Input: part model. Units: mm. Frame: model coordinates. Round coordinates to 2 decimals unless told otherwise and drop trailing zeros. Order: outer loops, then holes, each group sorted by start corner. A loop starts at its lowest first (then second) coordinate and runs counter-clockwise, first axis right, second up. Notation, with made-up numbers: (-9, -4.5) -> (13, -4.5) arc R35 ccw to (13, 32.5) -> close; hole circle Ø5 at (-17, -9.5). An arc over 180 degrees is marked (long way). Answer as CSV lines item,"result". Start each with the question number.
1) Section query C-C, the plane x = 17.5. Output: boundary loops of the cut face in (y, z), and give its area (3 significant figures).
2) Section query B-B, the plane z = 3.2. Output: boundary loops of the cut face in (x, y) (3 decimals).
3) Section query A-A, the plane y = -8.3. Output: boundary loops of the cut face in (x, z), and give its area (3 significant figures).
4) Line query: L1, parallel to Y at x = -12, z = 2.5; L2, parallel to Y at x = 15, z = 3.2; L3, parallel to X at y = 14.5, z = 1.3. Output: solid intervals per line, ascending.
```python
from build123d import *

# Parameters (mm, degrees)
SKETCH_1_W          = 42
SKETCH_1_H          = 42
EXTRUDE_1_DEPTH     = 5
SKETCH_2_R          = 1.275
CUT_EXTRUDE_1_DEPTH = 6
HOLE_WIZARD_M3_1_D  = 2.5


with BuildPart() as part:
    # 草图1 → 凸台-拉伸1 (new body)
    with BuildSketch(Plane.XY):
        Rectangle(SKETCH_1_W, SKETCH_1_H)
    extrude(amount=EXTRUDE_1_DEPTH)

    # 草图2 → 切除-拉伸1 (cut, through all)
    with BuildSketch(Plane.XY.offset(5)):
        with Locations((13.435028843, 13.435028843)):
            Circle(SKETCH_2_R)
        with Locations((13.435028843, -13.435028843)):
            Circle(SKETCH_2_R)
        with Locations((-13.435028843, -13.435028843)):
            Circle(SKETCH_2_R)
        with Locations((-13.435028843, 13.435028843)):
            Circle(SKETCH_2_R)
    extrude(amount=-CUT_EXTRUDE_1_DEPTH, mode=Mode.SUBTRACT)

    # M3 螺纹孔1 (through all)
    with Locations(Plane(origin=(21, 0, 0), x_dir=(0, 0, -1), z_dir=(1, 0, 0))):
        with Locations((-2.5, 8.3)):
            hole_wizard_m3_1 = Hole(HOLE_WIZARD_M3_1_D / 2)

    # 镜向1: M3 螺纹孔1 across plane
    add(hole_wizard_m3_1.mirror(Plane.ZX), mode=Mode.SUBTRACT)


solid = part.part
```
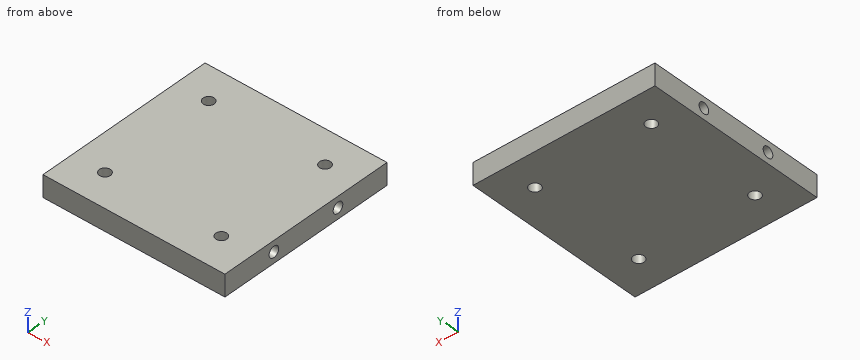
Findings:
1,outline,"(-21, 0) -> (21, 0) -> (21, 5) -> (-21, 5) -> close; hole circle Ø2.5 at (-8.3, 2.5); hole circle Ø2.5 at (8.3, 2.5)"
1,area,"200 mm^2"
2,outline,"(-21, -21) -> (21, -21) -> (21, -9.336) -> (-21, -9.336) -> close; (-21, -7.264) -> (21, -7.264) -> (21, 7.264) -> (-21, 7.264) -> close; (-21, 9.336) -> (21, 9.336) -> (21, 21) -> (-21, 21) -> close; hole circle Ø2.55 at (-13.435, -13.435); hole circle Ø2.55 at (-13.435, 13.435); hole circle Ø2.55 at (13.435, -13.435); hole circle Ø2.55 at (13.435, 13.435)"
3,outline,"(-21, 0) -> (21, 0) -> (21, 1.25) -> (-21, 1.25) -> close; (-21, 3.75) -> (21, 3.75) -> (21, 5) -> (-21, 5) -> close"
3,area,"105 mm^2"
4,L1,"y = -21 to -9.55, -7.05 to 7.05, 9.55 to 21"
4,L2,"y = -21 to -9.34, -7.26 to 7.26, 9.34 to 21"
4,L3,"x = -21 to -14.14, -12.73 to 12.73, 14.14 to 21"
